Study the drawing (mm; zero at the part's minimum x, y, z) and answer. Give positions to 0.01 mm unless a question says otherwise; leave off trailing zeros. Order: outer loops, then holes, each group sorted by start corner. A loop starts at its lowest first (then second) coordinate and runs counter-clockwise, first axis right, second up. Notation, with made-up numbers: (30, 41) - (59, 41) arc R17 cw to (59, 62) - close; hole circle Ø6 at (84.25, 22). An arc over 180 degrees is marked (long way). Return JSON: item names as keys, results as strings.
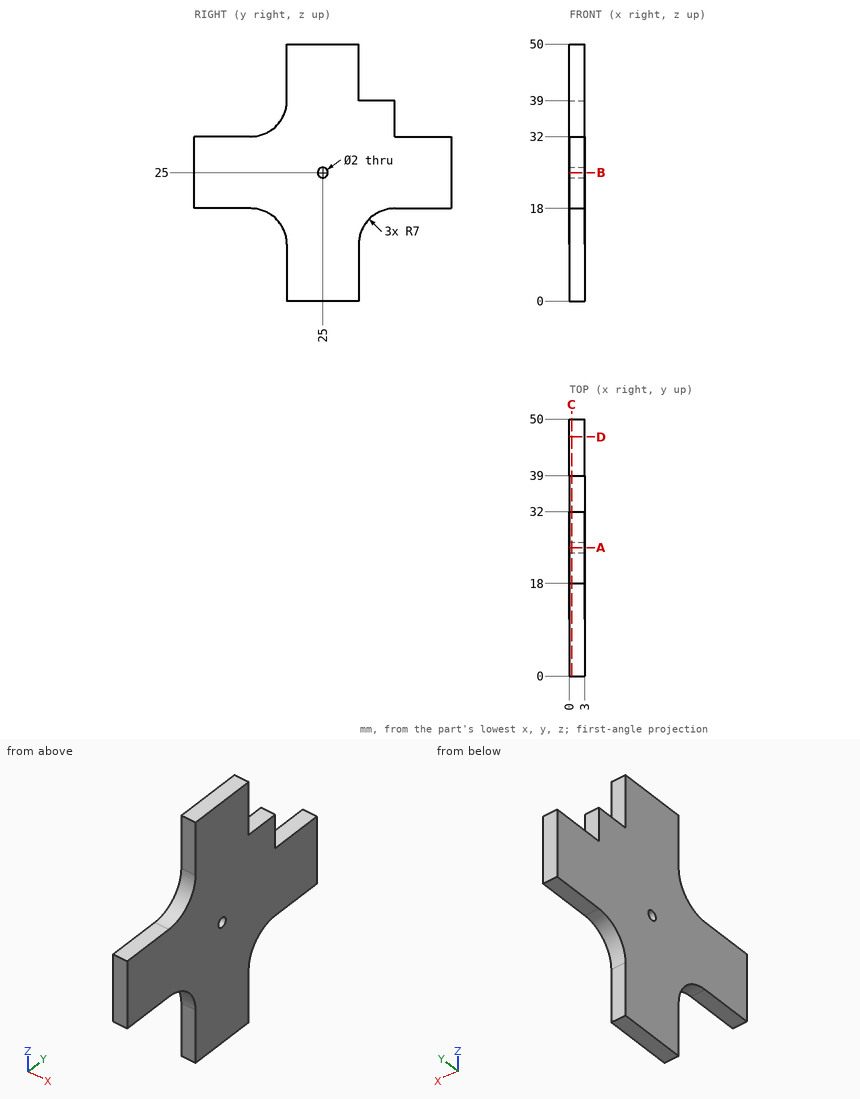
Q1. Given pin 1 (1.5 mm diameter, centred on x = 2, y = 45, fed in from -Z); pin 2 (0.9 mm diameter, centred on x = 1, z = 44, fed in from +Y); pin 3 (0.9 mm diameter, centred on x = 1.5, y = 44, fed in from +Z), each flat-ended and moving along its own axis, determine where each tip first touches the part or whether it passes through.
Values:
{"pin 1": "stops at z = 18", "pin 2": "stops at y = 32", "pin 3": "stops at z = 32"}
Q2. A cutting plane is placed at A-A (y = 25). Write down the section's boundary in (x, z), and give its area (3 significant figures).
Values:
{"outline": "(0, 0) - (3, 0) - (3, 24) - (0, 24) - close; (0, 26) - (3, 26) - (3, 50) - (0, 50) - close", "area": "144 mm²"}
Q3. Consider L1, parallel to Y at x = 1.1, z = 25; L2, parallel to Z at x = 1.55, y = 6. Determine where each line is inside the solid, lowest interval first.
Values:
{"L1": "y = 0 to 24, 26 to 50", "L2": "z = 18 to 32"}
Q4. A cutting plane is placed at D-D (y = 46.5). Write down the section's boundary in (x, z), and give its area (3 significant figures).
Values:
{"outline": "(0, 18) - (3, 18) - (3, 32) - (0, 32) - close", "area": "42.0 mm²"}
Q5. A cutting plane is placed at C-C (x = 0.45). Write down the section's boundary in (y, z).
Values:
{"outline": "(0, 18) - (11, 18) arc R7 cw to (18, 11) - (18, 0) - (32, 0) - (32, 11) arc R7 cw to (39, 18) - (50, 18) - (50, 32) - (39, 32) - (39, 39) - (32, 39) - (32, 50) - (18, 50) - (18, 39) arc R7 cw to (11, 32) - (0, 32) - close; hole circle Ø2 at (25, 25)"}
